The model under review builds one solid part; all positions refer to its coordinate system, in mm. Give positions to 0.01 mm unless a question says otherwise; leave off trailing zeros. Order: outer loops, then holes, each group sorted by start corner. A loop starts at its lowest first (then second) coordinate and runs counter-clockwise, first axis right, second up.
```python
from build123d import *

# Parameters (mm, degrees)
F0_W     = 19.05
F0_H     = 63.5
F1_DEPTH = 1257.3
F2_R     = 12.7
F3_DEPTH = 19.051


with BuildPart() as f1:
    # F0 (on Front) → F1 (new body)
    with BuildSketch(Plane.XZ):
        with Locations((9.525, -31.75)):
            Rectangle(F0_W, F0_H)
    extrude(amount=F1_DEPTH)

    # F2 (on face) → F3 (cut, through all)
    with BuildSketch(Plane.YZ.offset(19.05)):
        with Locations((-1104.9, -31.75)):
            Circle(F2_R)
        with Locations((-628.65, -31.75)):
            Circle(F2_R)
        with Locations((-152.4, -31.75)):
            Circle(F2_R)
    extrude(amount=-F3_DEPTH, mode=Mode.SUBTRACT)


solid = f1.part
```
Item 1: For line 1 (Y direction, x = 16.75, z = -32); line 2 (Y direction, x = 4.5, z = -33.5); line 3 (Z direction, x = 8.75, y = -628.65), list the stretches that pass through material, from the lowest coordinate up.
Values found:
line 1: y = -1257.3 to -1117.6, -1092.2 to -641.35, -615.95 to -165.1, -139.7 to 0
line 2: y = -1257.3 to -1117.48, -1092.32 to -641.23, -616.07 to -164.98, -139.82 to 0
line 3: z = -63.5 to -44.45, -19.05 to 0
Item 2: Clearance check with a flat-ended pin moving along its axis: pin 1 Ø8 at (x, z) = (13, -30.5) entering from +Y. State where the tip first meets the part, or that it passes through.
Values found:
pin 1: stops at y = 0
Item 3: Draft analysis for pull direction Y (two halves, no side actions). For faces 1 (the flat face through (9, 0, -31)), 2 (the flat face through (9, -1257.3, -31)), 3 (the cylindrical face through (9.658, -616.918, -36.614)), state which applies: released by +Y, released by -Y, zero draft, split by the parting line, or undercut.
Values found:
face 1: released by +Y
face 2: released by -Y
face 3: undercut
Item 4: Take a section at C-C (x = 4.75). Give the boundary of the cut face in (y, z).
Values found:
outline: (-1257.3, -63.5) - (0, -63.5) - (0, 0) - (-1257.3, 0) - close; hole circle Ø25.4 at (-1104.9, -31.75); hole circle Ø25.4 at (-628.65, -31.75); hole circle Ø25.4 at (-152.4, -31.75)
Item 5: Take a section at B-B (y = -1104.9). Give the boundary of the cut face in (x, z), and give its area (3 significant figures).
Values found:
outline: (0, -63.5) - (19.05, -63.5) - (19.05, -44.45) - (0, -44.45) - close; (0, -19.05) - (19.05, -19.05) - (19.05, 0) - (0, 0) - close
area: 726 mm2
Item 6: Take a section at A-A (z = -31.75). Give the boundary of the cut face in (x, y), and give its area (3 significant figures).
Values found:
outline: (0, -1257.3) - (19.05, -1257.3) - (19.05, -1117.6) - (0, -1117.6) - close; (0, -1092.2) - (19.05, -1092.2) - (19.05, -641.35) - (0, -641.35) - close; (0, -615.95) - (19.05, -615.95) - (19.05, -165.1) - (0, -165.1) - close; (0, -139.7) - (19.05, -139.7) - (19.05, 0) - (0, 0) - close
area: 22,500 mm2
